from build123d import *

# Parameters (mm, degrees)
SKETCH1_R           = 4.165
BOSS_EXTRUDE1_DEPTH = 3.1
SKETCH2_R           = 7
SKETCH2_R_2         = 4.165
BOSS_EXTRUDE3_DEPTH = 0.8
SKETCH4_R           = 9
SKETCH4_R_2         = 4.165
BOSS_EXTRUDE4_DEPTH = 2


with BuildPart() as part:
    # Sketch1 → Boss-Extrude1 (new body)
    with BuildSketch(Plane.XY):
        with BuildLine():
            Line((-60, 20), (60, 20))
            ThreePointArc((60, 20), (88.284271247, 8.284271247), (100, -20))
            Line((100, -20), (-100, -20))
            ThreePointArc((-100, -20), (-88.284271247, 8.284271247), (-60, 20))
        make_face()
        with Locations(Location((0, 8, 0), (0, 0, 180))):
            Circle(SKETCH1_R, mode=Mode.SUBTRACT)
        with Locations(Location((48, 8, 0), (0, 0, 180))):
            Circle(SKETCH1_R, mode=Mode.SUBTRACT)
        with Locations(Location((-48, 8, 0), (0, 0, 180))):
            Circle(SKETCH1_R, mode=Mode.SUBTRACT)
        with Locations(Location((-88.284271247, -10, 0), (0, 0, 180))):
            Circle(SKETCH1_R, mode=Mode.SUBTRACT)
        with Locations(Location((88.284271247, -10, 0), (0, 0, 180))):
            Circle(SKETCH1_R, mode=Mode.SUBTRACT)
    extrude(amount=BOSS_EXTRUDE1_DEPTH)

    # Sketch2 → Boss-Extrude3 (add)
    # profile 1 of 3: a face of its own
    with BuildSketch(Plane.XY.offset(3.1)):
        with Locations(Location((-48, 8, 0), (0, 0, 180))):
            Circle(SKETCH2_R)
        with Locations(Location((-48, 8, 0), (0, 0, 180))):
            Circle(SKETCH2_R_2, mode=Mode.SUBTRACT)
    # profile 2 of 3: a face of its own
    with BuildSketch(Plane.XY.offset(3.1)):
        with Locations(Location((0, 8, 0), (0, 0, 180))):
            Circle(SKETCH2_R)
        with Locations(Location((0, 8, 0), (0, 0, 180))):
            Circle(SKETCH2_R_2, mode=Mode.SUBTRACT)
    # profile 3 of 3: a face of its own
    with BuildSketch(Plane.XY.offset(3.1)):
        with Locations(Location((48, 8, 0), (0, 0, 180))):
            Circle(SKETCH2_R)
        with Locations(Location((48, 8, 0), (0, 0, 180))):
            Circle(SKETCH2_R_2, mode=Mode.SUBTRACT)
    extrude(amount=BOSS_EXTRUDE3_DEPTH)

    # Sketch4 → Boss-Extrude4 (add)
    # profile 1 of 2: a face of its own
    with BuildSketch(Plane.XY.offset(3.1)):
        with Locations(Location((-88.284271247, -10, 0), (0, 0, 180))):
            Circle(SKETCH4_R)
        with Locations(Location((-88.284271247, -10, 0), (0, 0, 180))):
            Circle(SKETCH4_R_2, mode=Mode.SUBTRACT)
    # profile 2 of 2: a face of its own
    with BuildSketch(Plane.XY.offset(3.1)):
        with Locations(Location((88.284271247, -10, 0), (0, 0, 180))):
            Circle(SKETCH4_R)
        with Locations(Location((88.284271247, -10, 0), (0, 0, 180))):
            Circle(SKETCH4_R_2, mode=Mode.SUBTRACT)
    extrude(amount=BOSS_EXTRUDE4_DEPTH)


solid = part.part
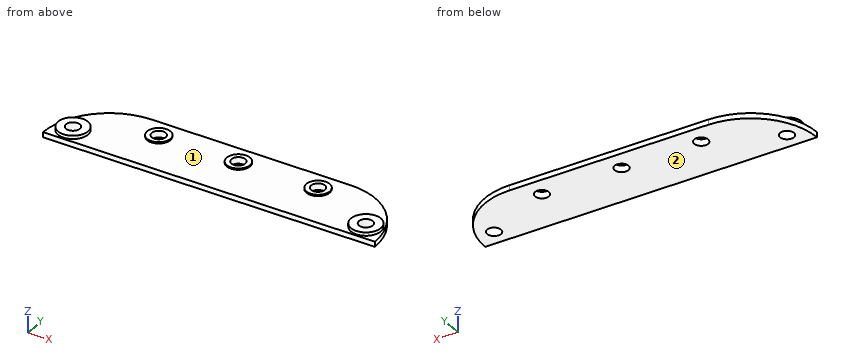
Design review of the part built by this model. Coordinates are the model's own, in mm. Face numbers are marked on the shaded views. Coordinates: 2 decimals unless noted, no trailing zeros. Loops run counter-clockwise (first coordinate to the right, second up) from the corner with the lowest first, then second, coordinate; pieces in that order, holes last.
Item 1: Wall thickness on L1, parallel to X at y = -7, z = 1.2; L2, parallel to X at y = 5, z = 1.5; L3, parallel to X at y = 8, z = 2.35 (3 decimals): over which ranges is each line inside the solid? List them lowest first.
Completed:
L1: x = -97.83 to -91.17, -85.4 to 85.4, 91.17 to 97.83
L2: x = -91.22 to -50.89, -45.11 to -2.89, 2.89 to 45.11, 50.89 to 91.22
L3: x = -88.566 to -52.165, -43.835 to -4.165, 4.165 to 43.835, 52.165 to 88.566
Item 2: Clearance check with flat-ended pins moving along their axes: pin 1 (9.5 mm diameter, centred on x = 88.28, y = -10, fed in from -Z); pin 2 (1.5 mm diameter, centred on y = -12.5, z = 4, fed in from +X); pin 3 (15.5 mm diameter, centred on x = 3, y = 11.5, fed in from +Z). State where each tip first meets the part, or that it passes through.
Completed:
pin 1: stops at z = 0
pin 2: stops at x = 97.11
pin 3: stops at z = 3.9
Item 3: Add section B-B (z = 1.3). Write out the cut boundary in (x, y) (3 decimals).
Completed:
outline: (-100, -20) - (100, -20) arc R40 ccw to (60, 20) - (-60, 20) arc R40 ccw to start; hole circle Ø8.33 at (-88.284, -10); hole circle Ø8.33 at (-48, 8); hole circle Ø8.33 at (0, 8); hole circle Ø8.33 at (48, 8); hole circle Ø8.33 at (88.284, -10)
Item 4: Add section C-C (y = -10). Write out the cut boundary in (x, z).
Completed:
outline: (-98.73, 0) - (-92.45, 0) - (-92.45, 5.1) - (-97.28, 5.1) - (-97.28, 3.1) - (-98.73, 3.1) - close; (-84.12, 0) - (84.12, 0) - (84.12, 5.1) - (79.28, 5.1) - (79.28, 3.1) - (-79.28, 3.1) - (-79.28, 5.1) - (-84.12, 5.1) - close; (92.45, 0) - (98.73, 0) - (98.73, 3.1) - (97.28, 3.1) - (97.28, 5.1) - (92.45, 5.1) - close
Item 5: Add section A-A (x = 48). Write out the cut boundary in (y, z) (3 decimals).
Completed:
outline: (-20, 0) - (3.835, 0) - (3.835, 3.9) - (1, 3.9) - (1, 3.1) - (-20, 3.1) - close; (12.165, 0) - (20, 0) - (20, 3.1) - (15, 3.1) - (15, 3.9) - (12.165, 3.9) - close
Item 6: Draft analysis for pull direction X (two halves, no side actions). For the marked faces 1 and 2, state which applies: pulls with the +X half, pulls with the -X half, needs draft (parallel to the pull), parting line crosses it, or undercut.
Completed:
face 1: undercut
face 2: needs draft
